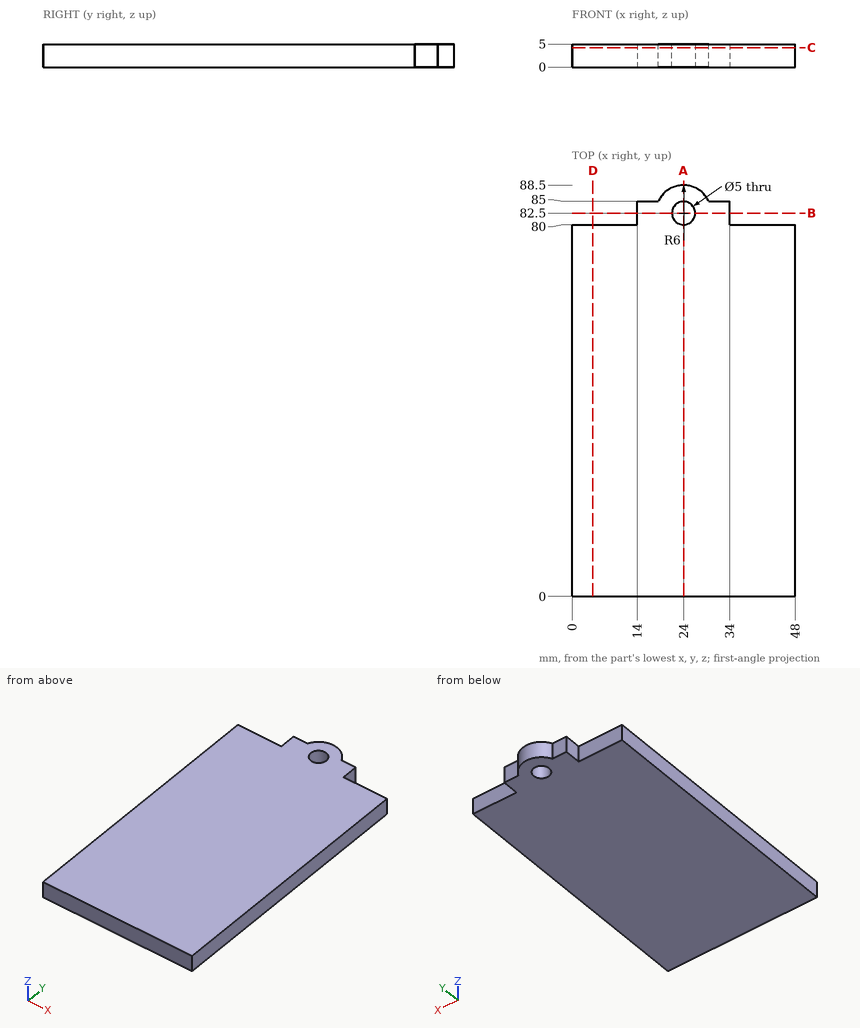
Part print with two shaded views. Sizes in mm from the minimum x, y, z corner. Round coordinates to 2 decimals unless told otherwise and drop trailing zeros. Order: outer loops, then holes, each group sorted by start corner. A loop starts at its lowest first (then second) coordinate and runs counter-clockwise, first axis right, second up. Notation, with made-up numbers: (7.25, 60.25) -> (31.25, 60.25) arc R23 cw to (31.25, 74.25) -> close; hole circle Ø9 at (-8.5, 55). An arc over 180 degrees is marked (long way). One line per question, with ' | ' between items.
Q1. Probe probe 1 along Y at (x, z) = (24, 3.15); probe 2 along Y at (x, z) = (40, 0.5); probe 3 along Y at (x, z) = (33.5, 1.05). List the from-to ranges inside material, lowest first.
Completed:
probe 1: y = 0 to 80, 85 to 88.5 | probe 2: y = 0 to 80 | probe 3: y = 0 to 85
Q2. Slice it at D-D (x = 4.5). Write the cut outline in (y, z).
Completed:
outline: (0, 0) -> (80, 0) -> (80, 5) -> (0, 5) -> close
Q3. Slice it at C-C (z = 4.2). Write the cut outline in (x, y), then the cut area to 3 significant figures.
Completed:
outline: (0, 0) -> (48, 0) -> (48, 80) -> (34, 80) -> (34, 85) -> (29.45, 85) arc R6 ccw to (18.55, 85) -> (14, 85) -> (14, 80) -> (0, 80) -> close; hole circle Ø5 at (24, 82.5) | area: 3,950 mm^2
Q4. Slice it at B-B (y = 82.5). Write the cut outline in (x, z), then the cut area to 3 significant figures.
Completed:
outline: (14, 0) -> (21.5, 0) -> (21.5, 5) -> (14, 5) -> close; (26.5, 0) -> (34, 0) -> (34, 5) -> (26.5, 5) -> close | area: 75.0 mm^2
Q5. Slice it at A-A (x = 24). Write the cut outline in (y, z), then the cut area to 4 significant figures.
Completed:
outline: (0, 0) -> (80, 0) -> (80, 5) -> (0, 5) -> close; (85, 0) -> (88.5, 0) -> (88.5, 5) -> (85, 5) -> close | area: 417.5 mm^2
Q6. Drop flat-ended pins along their axis: pin 1 (2.5 mm diameter, centred on x = 44, z = 2, fed in from +Y); pin 2 (2.5 mm diameter, centred on y = 81.5, z = 1.5, fed in from -X). Give the stop position or say it passes through.
Completed:
pin 1: stops at y = 80 | pin 2: stops at x = 14
